```python
from build123d import *

# Parameters (mm, degrees)
SKETCH1_W           = 241.3
SKETCH1_H           = 52.07
BOSS_EXTRUDE1_DEPTH = 3
SKETCH2_R           = 2
CUT_EXTRUDE1_DEPTH  = 124.463531964
SKETCH7_R           = 1.5
CUT_EXTRUDE3_DEPTH  = 124.463531964
SKETCH8_W           = 3
SKETCH8_H           = 52.07
CUT_EXTRUDE4_DEPTH  = 25.908


with BuildPart() as part:
    # Sketch1 → Boss-Extrude1 (new body)
    with BuildSketch(Plane.XY):
        Rectangle(SKETCH1_W, SKETCH1_H)
    extrude(amount=BOSS_EXTRUDE1_DEPTH)

    # Sketch2 → Cut-Extrude1 (cut, through all)
    with BuildSketch(Plane.XY.offset(3)):
        with Locations((113.339406907, 0)):
            Circle(SKETCH2_R)
        with Locations((-96.52, 0)):
            Circle(SKETCH2_R)
    extrude(amount=-CUT_EXTRUDE1_DEPTH, mode=Mode.SUBTRACT)

    # Sketch7 → Cut-Extrude3 (cut, through all)
    with BuildSketch(Plane.XY.offset(3)):
        with Locations((89.267430612, 0)):
            Circle(SKETCH7_R)
    extrude(amount=-CUT_EXTRUDE3_DEPTH, mode=Mode.SUBTRACT)

    # Sketch8 → Cut-Extrude4 (cut)
    with BuildSketch(Plane(origin=(120.65, 0, 0), x_dir=(0, 0, -1), z_dir=(1, 0, 0))):
        with Locations((-1.5, 0)):
            Rectangle(SKETCH8_W, SKETCH8_H)
    extrude(amount=-CUT_EXTRUDE4_DEPTH, mode=Mode.SUBTRACT)


solid = part.part
```
Geometry: final body of the model. Coordinates: model frame, mm. Coordinates: 2 decimals unless noted, no trailing zeros. Order: outer loops, then holes, each group sorted by start corner. A loop starts at its lowest first (then second) coordinate and runs counter-clockwise, first axis right, second up. Notation, with made-up numbers: (77.5, 14.5) - (87.5, 14.5) arc R14 cw to (87.5, 19.5) - close; hole circle Ø9 at (28, 33.25). An arc over 180 degrees is marked (long way). Write each question's results on one line, items separated by ' | '.
1) Pull-direction query (Y, two-part tool) for faces 1 (the cylindrical face through (-98.518, 0.088, 1.521)), 2 (the flat face through (-14, 0, 3)); classes: pulls with the +Y half, pulls with the -Y half, needs draft (parallel to the pull), parting line crosses it, or undercut.
Results list:
face 1: undercut | face 2: needs draft
2) Line query: line 1 (Y direction, x = -96.52, z = 1.7) (3 decimals). Output: solid intervals per line, ascending. Write a range as from..to.
Results list:
line 1: -26.035..-2, 2..26.035
3) Section A-A, the plane x = -96.52. Return loops of the section in (y, z) (3 decimals), plus the area to 3 significant figures.
Results list:
outline: (-26.035, 0) - (-2, 0) - (-2, 3) - (-26.035, 3) - close; (2, 0) - (26.035, 0) - (26.035, 3) - (2, 3) - close | area: 144 mm^2
4) Pin query (flat end, axial travel): pin 1 (4 mm diameter, centred on x = 89.27, y = 0, fed in from -Z). Return the tip coordinate at first contact, or that it passes through.
Results list:
pin 1: z = 0
